```python
from build123d import *

# Parameters (mm, degrees)
SKETCH1_W           = 130
SKETCH1_H           = 130
BOSS_EXTRUDE1_DEPTH = 40
FILLET1_R           = 3
SKETCH2_W           = 30.4
SKETCH2_H           = 30.4
CUT_EXTRUDE1_DEPTH  = 30
CHAMFER1_SIZE       = 1


with BuildPart() as part:
    # Sketch1 → Boss-Extrude1 (new body)
    with BuildSketch(Plane(origin=(0, 0, 0), x_dir=(1, 0, 0), z_dir=(0, 1, 0))):
        Rectangle(SKETCH1_W, SKETCH1_H)
    extrude(amount=BOSS_EXTRUDE1_DEPTH)

    # Fillet1
    fillet1_edges = [part.edges().sort_by_distance(p)[0] for p in [
        (65, 20, 65),
        (-65, 20, 65),
        (-65, 20, -65),
        (65, 20, -65),
    ]]
    fillet(fillet1_edges, radius=FILLET1_R)

    # Sketch2 → Cut-Extrude1 (cut)
    with BuildSketch(Plane(origin=(0, 40, 0), x_dir=(1, 0, 0), z_dir=(0, 1, 0))):
        Rectangle(SKETCH2_W, SKETCH2_H)
    extrude(amount=-CUT_EXTRUDE1_DEPTH, mode=Mode.SUBTRACT)

    # Chamfer1
    chamfer1_edges = [part.edges().sort_by_distance(p)[0] for p in [
        (15.2, 40, 0),
        (0, 40, -15.2),
        (-15.2, 40, 0),
        (0, 40, 15.2),
    ]]
    chamfer(chamfer1_edges, length=CHAMFER1_SIZE)


solid = part.part
```
Design review of the part built by this model. Coordinates are the model's own, in mm. A direction names the side the tool comes from. Give positions to 0.01 mm unless a question says otherwise; leave off trailing zeros. Write each loop counter-clockwise with the first axis right and the second up, starting at its lowest first coordinate (ties: lowest second). Pieces come first, ordered by that corner, then holes. Notation, with made-up numbers: (9.5, 72) - (28.5, 72) arc R6 cw to (28.5, 77) - close; hole circle Ø5 at (78.25, -35). An arc over 180 degrees is marked (long way). Return JSON: item names as keys, results as strings. Group by question number.
(1) We need section A-A, the plane y = 33.5. Give the boundary of the cut face in (x, z).
(2) Machinability: for faces 1 (the cylindrical face through (-64.14, 20.28, 64.1)), 2 (the flat face through (0, 25, 15.2)), which of the approach directions +Z, -Z, +X, -X, +Y, -Y give a long, thin tool a straight path to every point of the face, cutting with its end or side? Answer none if there is none.
(3) We need section B-B, the plane z = 8. Give the boundary of the cut face in (x, y).
(4) Mouldability with a two-part tool opening along X and no side actions: class faces 3 (the cylindrical face through (-64.14, 20.28, -64.1)), 4 (the flat face through (0, 10, 0)), 5 (the flat face through (-1, 20, -65)) as +X half, -X half, draft (parallel to the pull), parting line (faces both ways), or undercut.
(5) To check wall thickness, follow probe 1 along X at (y, z) = (14, 3.5). State the ranges of the line that lie inside material, in increasing order.
Reported:
{
 "1": {"outline": "(-65, -62) arc R3 ccw to (-62, -65) - (62, -65) arc R3 ccw to (65, -62) - (65, 62) arc R3 ccw to (62, 65) - (-62, 65) arc R3 ccw to (-65, 62) - close; hole (-15.2, -15.2) - (15.2, -15.2) - (15.2, 15.2) - (-15.2, 15.2) - close"},
 "2": {"face 1": "+Z, -X, +Y, -Y", "face 2": "+Y"},
 "3": {"outline": "(-65, 0) - (65, 0) - (65, 40) - (16.2, 40) - (15.2, 39) - (15.2, 10) - (-15.2, 10) - (-15.2, 39) - (-16.2, 40) - (-65, 40) - close"},
 "4": {"face 3": "-X half", "face 4": "undercut", "face 5": "draft"},
 "5": {"probe 1": "x = -65 to -15.2, 15.2 to 65"}
}
